CAD build for the part. Positions are in the model's coordinates, mm. A direction names the side the tool comes from. Give positions to 0.01 mm unless a question says otherwise; leave off trailing zeros. Order: outer loops, then holes, each group sorted by start corner. A loop starts at its lowest first (then second) coordinate and runs counter-clockwise, first axis right, second up.
from build123d import *

# Parameters (mm, degrees)
F1_DEPTH  = 19.05
F3_DEPTH  = 12.7
F4_R      = 11.1125
F5_DEPTH  = 35.71748
F6_R      = 11.1125
F7_DEPTH  = 42.46626
F8_R      = 10.3505
F9_DEPTH  = 0.7874
F10_R     = 10.3505
F11_DEPTH = 0.7874
F12_R     = 11.1125
F13_DEPTH = 45.24248
F14_R     = 10.3505
F15_DEPTH = 0.7874
F16_R     = 11.1125
F17_DEPTH = 4.7752
F18_R     = 1.524
F19_R     = 11.1125
F20_DEPTH = 45.24248
F21_R     = 10.3505
F22_DEPTH = 0.7874
F23_R     = 11.1125
F24_DEPTH = 4.7752
F25_SIZE  = 3.175


with BuildPart() as f1:
    # F0 (on Right) → F1 (new body, symmetric)
    with BuildSketch(Plane.YZ):
        with BuildLine():
            Line((7.9375, -5.2651418547), (7.9375, 5.2651418547))
            ThreePointArc((7.9375, 5.2651418547), (0, 9.525), (-7.9375, 5.2651418547))
            Line((-7.9375, 5.2651418547), (-7.9375, -5.2651418547))
            ThreePointArc((-7.9375, -5.2651418547), (0, -9.525), (7.9375, -5.2651418547))
        make_face()
    extrude(amount=F1_DEPTH, both=True)

    # F2 (on face) → F3 (join)
    with BuildSketch(Plane.YZ.offset(19.05)):
        with BuildLine():
            Line((-7.9375, 7.7771299333), (-7.9375, -7.7771299333))
            ThreePointArc((-7.9375, -7.7771299333), (0, -11.1125), (7.9375, -7.7771299333))
            Line((7.9375, -7.7771299333), (7.9375, 7.7771299333))
            ThreePointArc((7.9375, 7.7771299333), (0, 11.1125), (-7.9375, 7.7771299333))
        make_face()
    extrude(amount=F3_DEPTH)

    # F4 (on face) → F5 (join)
    with BuildSketch(Plane.YZ.offset(31.75)):
        Circle(F4_R)
    extrude(amount=F5_DEPTH)

    # F6 (on face) → F7 (join)
    with BuildSketch(Plane(origin=(-19.05, 0, 0), x_dir=(0, -1, 0), z_dir=(-1, 0, 0))):
        Circle(F6_R)
    extrude(amount=F7_DEPTH)

    # F8 (on face) → F9 (join)
    with BuildSketch(Plane.YZ.offset(67.46748)):
        Circle(F8_R)
    extrude(amount=F9_DEPTH)

    # F10 (on face) → F11 (join)
    with BuildSketch(Plane(origin=(-61.51626, 0, 0), x_dir=(0, -1, 0), z_dir=(-1, 0, 0))):
        Circle(F10_R)
    extrude(amount=F11_DEPTH)

    # F12 (on face) → F13 (join)
    with BuildSketch(Plane(origin=(-62.30366, 0, 0), x_dir=(0, -1, 0), z_dir=(-1, 0, 0))):
        Circle(F12_R)
    extrude(amount=F13_DEPTH)

    # F14 (on face) → F15 (join)
    with BuildSketch(Plane(origin=(-107.54614, 0, 0), x_dir=(0, -1, 0), z_dir=(-1, 0, 0))):
        Circle(F14_R)
    extrude(amount=F15_DEPTH)

    # F16 (on face) → F17 (join)
    with BuildSketch(Plane(origin=(-108.33354, 0, 0), x_dir=(0, -1, 0), z_dir=(-1, 0, 0))):
        Circle(F16_R)
    extrude(amount=F17_DEPTH)

    # F18
    f18_edges = [f1.edges().sort_by_distance(p)[0] for p in [
        (-113.10874, 11.1125, 0),
    ]]
    fillet(f18_edges, radius=F18_R)

    # F19 (on face) → F20 (join)
    with BuildSketch(Plane.YZ.offset(68.25488)):
        Circle(F19_R)
    extrude(amount=F20_DEPTH)

    # F21 (on face) → F22 (join)
    with BuildSketch(Plane.YZ.offset(113.49736)):
        Circle(F21_R)
    extrude(amount=F22_DEPTH)

    # F23 (on face) → F24 (join)
    with BuildSketch(Plane.YZ.offset(114.28476)):
        Circle(F23_R)
    extrude(amount=F24_DEPTH)

    # F25
    f25_edges = [f1.edges().sort_by_distance(p)[0] for p in [
        (119.05996, -11.1125, 0),
    ]]
    chamfer(f25_edges, length=F25_SIZE)


solid = f1.part
1. 3-axis set-ups, long thin cutter, end or side, ignore diameter. For faces 1 (the cylindrical face through (0.267, 0.131, 9.524)), 2 (the cylindrical face through (-61.9, 8.21, -6.3)), 3 (the flat face through (6, 7.938, 0)), 4 (the cylindrical face through (-109.94, -10.6, 3.34)), 5 (the flat face through (6, -7.938, 0)): which of +Z, -Z, +X, -X, +Y, -Y reach the whole face in a straight line?
2. Mould opens along X. For faces 6 (the flat face through (19.05, 0, -10)), 7 (the cylindrical face through (115.07, 10.6, 3.34)), 8 (the flat face through (119.06, 0, 0)) say: released by +X, released by -X, zero draft, split by the parting line, or undercut.
3. Pin check, flat tips, straight feed: P1, Ø1, axis at x = 3, z = -3, coming from the -Y side; P2, Ø1, axis at x = 49.5, z = -2.5, coming from the +Y side; P3, Ø6, axis at x = 2, y = -4, coming from the -Z side. Stop position of each tip, or through.
4. Wall check: line 1 (Z direction, x = -79.5, y = -0.75); line 2 (Y direction, x = -8, z = -5.5); line 3 (Y direction, x = 94, z = -1). Give the ranges that are in metal, low to high.
5. Saw through at A-A on x = 79. Give the cut face in (y, z) (1 decimal).
Reported:
1. face 1: +Z
1. face 2: none
1. face 3: +Z, -Z, +Y
1. face 4: +X, -X
1. face 5: +Z, -Z, -Y
2. face 6: undercut
2. face 7: zero draft
2. face 8: released by +X
3. P1: stops at y = -7.94
3. P2: stops at y = 10.93
3. P3: stops at z = -9.47
4. line 1: z = -11.09 to 11.09
4. line 2: y = -7.78 to 7.78
4. line 3: y = -11.07 to 11.07
5. outline: circle Ø22.2 at (0, 0)
